```python
from build123d import *

# Parameters (mm, degrees)
F0_R     = 45
F0_R_2   = 2
F1_DEPTH = 9
F2_DEPTH = 7
F3_DEPTH = 2


with BuildPart() as f1:
    # F0 (on Top) → F1 (new body)
    with BuildSketch(Plane.XY):
        Circle(F0_R)
        with Locations((-38.351216, -14.497732)):
            Circle(F0_R_2, mode=Mode.SUBTRACT)
        with Locations((6.5625, -3.630922)):
            Circle(F0_R_2, mode=Mode.SUBTRACT)
        with Locations((38.351216, -14.497732)):
            Circle(F0_R_2, mode=Mode.SUBTRACT)
        Circle(F0_R_2, mode=Mode.SUBTRACT)
        with Locations((0, 41)):
            Circle(F0_R_2, mode=Mode.SUBTRACT)
        with Locations((6.5625, -3.630922)):
            Circle(F0_R_2)
    extrude(amount=-F1_DEPTH)

    # F0 (on Top) → F2 (join)
    with BuildSketch(Plane.XY):
        Circle(F0_R_2)
        with Locations((0, 41)):
            Circle(F0_R_2)
        with Locations((38.351216, -14.497732)):
            Circle(F0_R_2)
        with Locations((-38.351216, -14.497732)):
            Circle(F0_R_2)
    extrude(amount=-F2_DEPTH)

    # F0 (on Top) → F3 (cut)
    with BuildSketch(Plane.XY):
        with Locations((6.5625, -3.630922)):
            Circle(F0_R_2)
    extrude(amount=-F3_DEPTH, mode=Mode.SUBTRACT)


solid = f1.part
```
Work out the finished part from the listing and answer in its coordinate system (mm). A direction names the side the tool comes from. Round coordinates to 2 decimals unless told otherwise and drop trailing zeros. Loops run counter-clockwise (first coordinate to the right, second up) from the corner with the lowest first, then second, coordinate; pieces in that order, holes last. Notation, with made-up numbers: M 45.5,-22 L 56.5,-22 A14 ccw 56.5,-5 Z; hole C 59.25,-30 d11. An arc over 180 degrees is marked long. Use CSV: the item, a comma, the result in double quotes.
Q1. Each of these flat-tipped pins is pushed along its axis until it touches: pin 1 (2 mm diameter, centred on x = -38.5, y = -15, fed in from -Z); pin 2 (2 mm diameter, centred on x = 6, y = -3, fed in from +Z); pin 3 (3 mm diameter, centred on x = -9, z = -1, fed in from -Y). Where does it stop, or does it pass through?
Determined:
pin 1,"z = -7"
pin 2,"z = -2"
pin 3,"y = -44.37"
Q2. Section B-B, the plane y = 41 is taken. Determine the outline of the cut face in (x, z).
Determined:
outline,"M -18.55,-9 L -2,-9 L -2,-7 L 2,-7 L 2,-9 L 18.55,-9 L 18.55,0 L -18.55,0 Z"
Q3. Section D-D, the plane x = 20.5 is taken. Determine the outline of the cut face in (y, z), then the cut area to 3 significant figures.
Determined:
outline,"M -40.06,-9 L 40.06,-9 L 40.06,0 L -40.06,0 Z"
area,"721 mm2"
Q4. Section C-C, the plane z = -3.25 is taken. Determine the outline of the cut face in (x, y).
Determined:
outline,"C 0,0 d90"
Q5. Section A-A, the plane x = 0 is taken. Determine the outline of the cut face in (y, z).
Determined:
outline,"M -45,-9 L -2,-9 L -2,-7 L 2,-7 L 2,-9 L 39,-9 L 39,-7 L 43,-7 L 43,-9 L 45,-9 L 45,0 L -45,0 Z"
Q6. Consider L1, parallel to Y at x = 0, z = -8.05; L2, parallel to Y at x = -19, z = -3.25; L3, parallel to X at y = -25, z = -4.5. Determine where each line is inside the solid, lowest interval first.
Determined:
L1,"-45 to -2, 2 to 39, 43 to 45"
L2,"-40.79 to 40.79"
L3,"-37.42 to 37.42"
Q7. The mould has two halves that part along Y. Classify faces 1 (the flat face through (-1, 1, 0)), 2 (the flat face through (38, -14, -7)), 3 (the flat face through (7, -4, -2)), 4 (the cylindrical face through (20.765, -39.923, -4.437)): pulls with the +Y half, pulls with the -Y half, needs draft (parallel to the pull), parting line crosses it, or undercut.
Determined:
face 1,"needs draft"
face 2,"undercut"
face 3,"undercut"
face 4,"parting line crosses it"
Q8. A tool of negligible diameter and unlimited length cuts with its end or side. For faces 5 (the cylindrical face through (40.2, -15.26, -7.99)), 6 (the cylindrical face through (5.09, -2.28, -0.99)), 7 (the flat face through (-1, -9, -9)), from which of +Z, -Z, +X, -X, +Y, -Y can it reach the whole face along a straight path? Write none if from no direction.
Determined:
face 5,"-Z"
face 6,"+Z"
face 7,"-Z, +X, -X, +Y, -Y"
